The figure shows three views and two pictorial views of one solid part (mm, origin at its lowest corner). Answer the questions. A direction names the side the tool comes from. Give positions to 0.01 mm unless a question says otherwise; leave off trailing zeros. Write each loop counter-clockwise with the first axis right and the second up, starting at its lowest first coordinate (ties: lowest second). Pieces come first, ordered by that corner, then holes. Notation, with made-up numbers: M 69,2 L 111,2 A36 ccw 111,36 Z; hole C 21,39 d6. An arc over 180 degrees is marked long. Return JSON: item names as keys, results as strings.
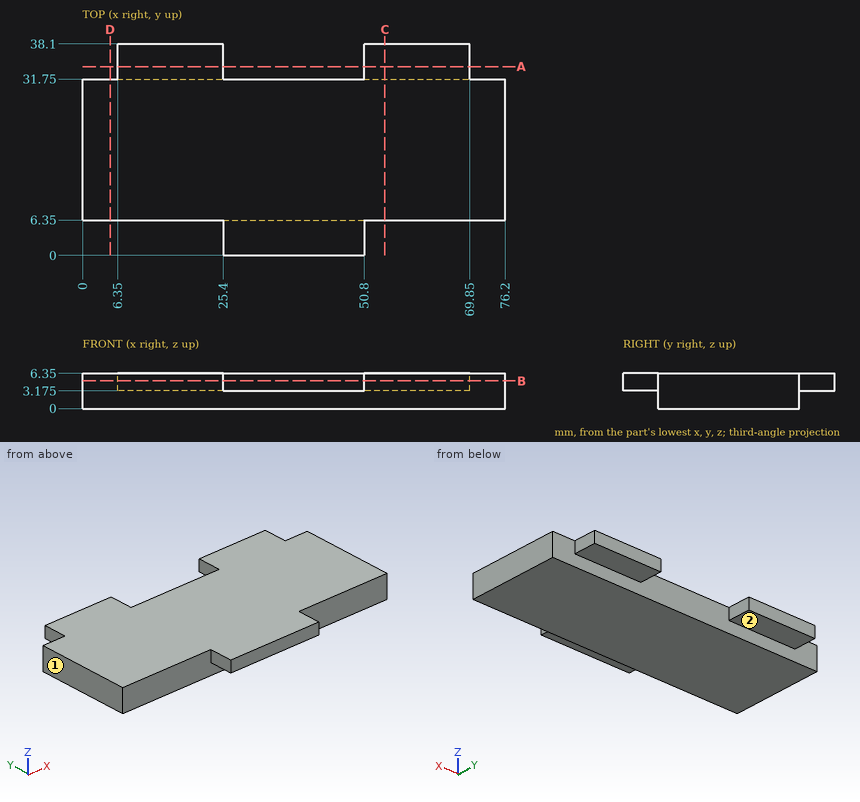
Item 1: A cutting plane is placed at A-A, the plane y = 34. Write down the section's boundary in (x, z) (3 decimals).
Geometry results:
{"outline": "M 6.35,3.175 L 25.4,3.175 L 25.4,6.35 L 6.35,6.35 Z; M 50.8,3.175 L 69.85,3.175 L 69.85,6.35 L 50.8,6.35 Z"}
Item 2: Which of the six approach directions +Z, -Z, +X, -X, +Y, -Y give full straight-line access (tool end or side, diameter ignored) to the marked faces 1 and 2?
Geometry results:
{"face 1": "+Z, -Z, -X, +Y, -Y", "face 2": "-Z, +X, -X, +Y"}
Item 3: Find the intervals of material crossed by line 1 (X direction, y = 35, z = 5.5); line 2 (Y direction, x = 8, z = 1.5); line 3 (Y direction, x = 21, z = 3.5), in increasing order.
Geometry results:
{"line 1": "x = 6.35 to 25.4, 50.8 to 69.85", "line 2": "y = 6.35 to 31.75", "line 3": "y = 6.35 to 38.1"}
Item 4: A cutting plane is placed at B-B, the plane z = 5. Write down the section's boundary in (x, y).
Geometry results:
{"outline": "M 0,6.35 L 25.4,6.35 L 25.4,0 L 50.8,0 L 50.8,6.35 L 76.2,6.35 L 76.2,31.75 L 69.85,31.75 L 69.85,38.1 L 50.8,38.1 L 50.8,31.75 L 25.4,31.75 L 25.4,38.1 L 6.35,38.1 L 6.35,31.75 L 0,31.75 Z"}
Item 5: A cutting plane is placed at D-D, the plane x = 5. Write down the section's boundary in (y, z).
Geometry results:
{"outline": "M 6.35,0 L 31.75,0 L 31.75,6.35 L 6.35,6.35 Z"}
Item 6: Given pin 1 Ø3.5 at (y, z) = (3, 5) entering from +X; pin 2 Ø1 at (y, z) = (34, 4.5) entering from +X; pin 3 Ø2.5 at (y, z) = (3, 4.5) entering from -X, each flat-ended and moving along its own axis, determine where each tip first touches the part or whether it passes through.
Geometry results:
{"pin 1": "stops at x = 50.8", "pin 2": "stops at x = 69.85", "pin 3": "stops at x = 25.4"}
Item 7: A cutting plane is placed at C-C, the plane x = 54.5. Write down the section's boundary in (y, z) (3 decimals).
Geometry results:
{"outline": "M 6.35,0 L 31.75,0 L 31.75,3.175 L 38.1,3.175 L 38.1,6.35 L 6.35,6.35 Z"}
